Verification items for the finished model (mm, model axes). Face numbers are marked on the shaded views. Round coordinates to 2 decimals unless told otherwise and drop trailing zeros. Write each loop counter-clockwise with the first axis right and the second up, starting at its lowest first coordinate (ties: lowest second). Pieces come first, ordered by that corner, then holes. Notation, with made-up numbers: M 51.25,53.5 L 79.25,53.5 A32 cw 79.25,84.5 Z; hole C -17,-19.5 d4. An arc over 180 degrees is marked long. One line per question, with ' | ' between items. Start each with the question number.
Q1. Cross-section at D-D (y = 40.4). Record the boundary of the cut face in (x, z) (3 decimals).
Q2. Release check for a two-part mould opening along X. For the marked faces 1 and 2 record: released by +X, released by -X, zero draft, split by the parting line, or undercut.
Q3. Cross-section at C-C (x = -1). Record the boundary of the cut face in (y, z) (3 decimals).
Q4. Thickness scan on line 1 along Y through (x, z) = (17.5, -0.9); line 2 along Y through (x, z) = (17.5, -0.8); line 3 along Z through (x, y) = (-6, 38.5) (3 decimals). Record the ranges inside material, lowest first. Write a range as from..to.
Q5. Cross-section at B-B (y = 23.5). Record the boundary of the cut face in (x, z) (3 decimals).
Q6. Cross-section at A-A (x = -17.5). Record the boundary of the cut face in (y, z) (3 decimals).
Q7. Gauge pin test, flat ends, axial feed: pin 1 (3 mm diameter, centred on y = 38.5, z = 2.5, fed in from +X); pin 2 (12.5 mm diameter, centred on x = -1.5, y = 28.5, fed in from +Z) (3 decimals); pin 3 (4 mm diameter, centred on x = -11.5, z = 4, fed in from -Y). Record the tip position at first contact, or that the pin passes through.
from build123d import *

# Parameters (mm, degrees)
SKETCH1_W            = 44.8
SKETCH1_H            = 2.99
BOSS_EXTRUDE1_DEPTH  = 44.8
FILLET1_RADIUS       = 1.495
FILLET1_LENGTH       = 44.8
M4_CLEARANCE_HOLE1_D = 4.8
M3_CLEARANCE_HOLE1_D = 3.4
SKETCH8_R            = 1.7
BOSS_EXTRUDE2_DEPTH  = 4
REVOLVE1_ANGLE       = 180
REVOLVE2_ANGLE       = 180
FILLET2_RADIUS       = 1.495
FILLET2_LENGTH       = 44.8
FILLET3_R            = 1
FILLET4_R            = 1


with BuildPart() as part:
    # Sketch1 → Boss-Extrude1 (new body)
    with BuildSketch(Plane(origin=(0, 0, 0), x_dir=(1, 0, 0), z_dir=(0, 1, 0))):
        Rectangle(SKETCH1_W, SKETCH1_H)
    extrude(amount=BOSS_EXTRUDE1_DEPTH)

    # Fillet1: full round fillet: the end face becomes a half cylinder, R = half its width
    fillet1_face = Plane((0, 0, 0), x_dir=(-1, 0, 0), z_dir=(0, -1, 0))  # on the end face: x along it, z out of the body
    fillet1_slab = fillet1_face.offset(-FILLET1_RADIUS / 2) * Box(FILLET1_LENGTH, 2 * FILLET1_RADIUS, FILLET1_RADIUS, mode=Mode.PRIVATE)  # the body's end, R deep
    fillet1_round = Plane((0, 1.495, 0), x_dir=(0, -1, 0), z_dir=(-1, 0, 0)) * Cylinder(FILLET1_RADIUS, FILLET1_LENGTH, mode=Mode.PRIVATE)  # its axis R under the face
    add(fillet1_slab - fillet1_round, mode=Mode.SUBTRACT)

    # M4 Clearance Hole1 (through all)
    with Locations(Plane.XY.offset(1.495)):
        with Locations((-17.5, 40.4), (-17.5, 20.4), (17.5, 20.4), (17.5, 40.4)):
            Hole(M4_CLEARANCE_HOLE1_D / 2)

    # M3 Clearance Hole1 (through all)
    with Locations(Plane.XY.offset(1.495)):
        with Locations((0, 8.2)):
            Hole(M3_CLEARANCE_HOLE1_D / 2)

    # Sketch8 → Boss-Extrude2 (add)
    with BuildSketch(Plane.XY.offset(1.495)):
        with Locations(Location((-10.5, 8.2, 0), (0, 0, 180))):
            Circle(SKETCH8_R)
        with Locations(Location((10.5, 8.2, 0), (0, 0, 180))):
            Circle(SKETCH8_R)
    extrude(amount=BOSS_EXTRUDE2_DEPTH)

    # Sketch9 → Revolve1 (revolve)
    with BuildSketch(Plane.XY.offset(5.495)):
        with BuildLine():
            Line((-10.5, 9.9), (-10.5, 6.5))
            ThreePointArc((-10.5, 6.5), (-8.8, 8.2), (-10.5, 9.9))
        make_face()
    revolve(axis=Axis((-10.5, 9.9, 5.495), (0, -1, 0)), revolution_arc=REVOLVE1_ANGLE)

    # Sketch10 → Revolve2 (revolve)
    with BuildSketch(Plane.XY.offset(5.495)):
        with BuildLine():
            Line((10.5, 9.9), (10.5, 6.5))
            ThreePointArc((10.5, 6.5), (12.2, 8.2), (10.5, 9.9))
        make_face()
    revolve(axis=Axis((10.5, 9.9, 5.495), (0, -1, 0)), revolution_arc=REVOLVE2_ANGLE)

    # Fillet2: full round fillet: the end face becomes a half cylinder, R = half its width
    fillet2_face = Plane((0, 44.8, 0), x_dir=(1, 0, 0), z_dir=(0, 1, 0))  # on the end face: x along it, z out of the body
    fillet2_slab = fillet2_face.offset(-FILLET2_RADIUS / 2) * Box(FILLET2_LENGTH, 2 * FILLET2_RADIUS, FILLET2_RADIUS, mode=Mode.PRIVATE)  # the body's end, R deep
    fillet2_round = Plane((0, 43.305, 0), x_dir=(0, 1, 0), z_dir=(1, 0, 0)) * Cylinder(FILLET2_RADIUS, FILLET2_LENGTH, mode=Mode.PRIVATE)  # its axis R under the face
    add(fillet2_slab - fillet2_round, mode=Mode.SUBTRACT)

    # Fillet3
    fillet3_edges = [part.edges().sort_by_distance(p)[0] for p in [
        (-22.4, 0, 0),
        (-22.4, 22.4, 1.495),
        (-22.4, 22.4, -1.495),
        (-22.4, 44.8, 0),
    ]]
    fillet(fillet3_edges, radius=FILLET3_R)

    # Fillet4
    fillet4_edges = [part.edges().sort_by_distance(p)[0] for p in [
        (22.4, 0, 0),
        (22.4, 22.4, 1.495),
        (22.4, 22.4, -1.495),
        (22.4, 44.8, 0),
    ]]
    fillet(fillet4_edges, radius=FILLET4_R)


solid = part.part
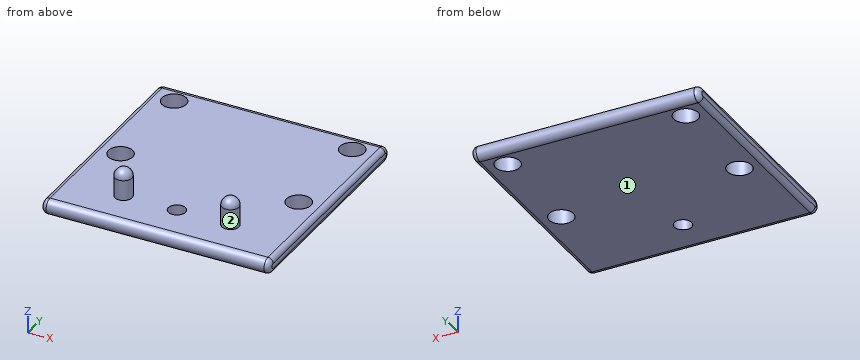
Determined:
1) outline: M -22.4,-0.495 A1 ccw -21.4,-1.495 L -19.9,-1.495 L -19.9,1.495 L -21.4,1.495 A1 ccw -22.4,0.495 Z; M -15.1,-1.495 L 15.1,-1.495 L 15.1,1.495 L -15.1,1.495 Z; M 19.9,-1.495 L 21.4,-1.495 A1 ccw 22.4,-0.495 L 22.4,0.495 A1 ccw 21.4,1.495 L 19.9,1.495 Z
2) face 1: zero draft | face 2: undercut
3) outline: M 1.495,-1.495 L 6.825,-1.495 L 6.825,1.495 L 1.495,1.495 A1.495 ccw Z; M 9.575,-1.495 L 43.305,-1.495 A1.495 ccw 43.305,1.495 L 9.575,1.495 Z
4) line 1: y = 0.3..18, 22.8..38, 42.8..44.5 | line 2: y = 0.23..18, 22.8..38, 42.8..44.57 | line 3: z = -1.495..1.495
5) outline: M -22.4,-0.495 A1 ccw -21.4,-1.495 L 21.4,-1.495 A1 ccw 22.4,-0.495 L 22.4,0.495 A1 ccw 21.4,1.495 L -21.4,1.495 A1 ccw -22.4,0.495 Z
6) outline: M 1.495,-1.495 L 18,-1.495 L 18,1.495 L 1.495,1.495 A1.495 ccw Z; M 22.8,-1.495 L 38,-1.495 L 38,1.495 L 22.8,1.495 Z; M 42.8,-1.495 L 43.305,-1.495 A1.495 ccw 43.305,1.495 L 42.8,1.495 Z
7) pin 1: stops at x = 22.26 | pin 2: stops at z = 1.495 | pin 3: stops at y = 6.5
